Read the model definition and answer for the solid it produces. Units are mm, in the model's axes. Face numbers are marked on the shaded views. A direction names the side the tool comes from. Coordinates: 2 decimals unless noted, no trailing zeros. Write each loop counter-clockwise with the first axis right and the second up, starting at its lowest first coordinate (ties: lowest second). Pieces come first, ordered by that corner, then holes.
1) Each of these flat-tipped pins is pushed along its axis until it touches: pin 1 Ø8 at (y, z) = (25.5, 10.5) entering from +X; pin 2 Ø4 at (x, z) = (21.5, 3.5) entering from +Y; pin 3 Ø4 at (x, y) = (10, 4) entering from -Z. Where does it stop, or does it pass through?
2) The part is cut by section D-D (y = -18). Determine the outline of the cut face in (x, z).
3) Which of the six approach directions +Z, -Z, +X, -X, +Y, -Y give full straight-line access (tool end or side, diameter ignored) to the marked faces 1 and 2?
4) The part is cut by section C-C (x = 24.5). Determine the outline of the cut face in (y, z), then the cut area to 3 significant figures.
5) Find the intervals of material crossed by line 1 (Z direction, x = 20, y = 0); line 2 (Z direction, x = 34.5, y = 0); line 3 (X direction, y = -20, z = 4), in increasing order.
6) The part is cut by section A-A (y = 0). Determine the outline of the cut face in (x, z), then the cut area to 3 significant figures.
from build123d import *

# Parameters (mm, degrees)
F0_R     = 31.75
F1_DEPTH = 25.4
F2_R     = 19.05
F3_DEPTH = 44.45
F4_R     = 12.7
F5_DEPTH = 44.45


with BuildPart() as f1:
    # F0 (on Right) → F1 (new body)
    with BuildSketch(Plane.YZ):
        Circle(F0_R)
    extrude(amount=F1_DEPTH)

    # F2 (on Right) → F3 (join)
    with BuildSketch(Plane.YZ):
        Circle(F2_R)
    extrude(amount=F3_DEPTH)

    # F4 (on Right) → F5 (cut)
    with BuildSketch(Plane.YZ):
        Circle(F4_R)
    extrude(amount=F5_DEPTH, mode=Mode.SUBTRACT)


solid = f1.part
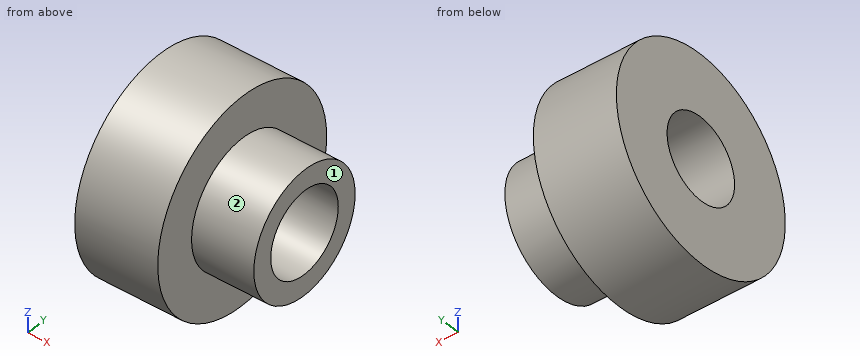
Reported:
1. pin 1: stops at x = 25.4
1. pin 2: stops at y = 31.71
1. pin 3: stops at z = -31.69
2. outline: (0, -26.15) - (25.4, -26.15) - (25.4, -6.24) - (44.45, -6.24) - (44.45, 6.24) - (25.4, 6.24) - (25.4, 26.15) - (0, 26.15) - close
3. face 1: +Z, -Z, +X, +Y, -Y
3. face 2: +X
4. outline: circle Ø63.5 at (0, 0); hole circle Ø25.4 at (0, 0)
4. area: 2,660 mm2
5. line 1: z = -31.75 to -12.7, 12.7 to 31.75
5. line 2: z = -19.05 to -12.7, 12.7 to 19.05
5. line 3: x = 0 to 25.4
6. outline: (0, -31.75) - (25.4, -31.75) - (25.4, -19.05) - (44.45, -19.05) - (44.45, -12.7) - (0, -12.7) - close; (0, 12.7) - (44.45, 12.7) - (44.45, 19.05) - (25.4, 19.05) - (25.4, 31.75) - (0, 31.75) - close
6. area: 1,210 mm2
